Here's how the part is built. I have some questions about the finished solid (model axes, mm). A direction names the side the tool comes from. Coordinates: 2 decimals unless noted, no trailing zeros. Write each loop counter-clockwise with the first axis right and the second up, starting at its lowest first coordinate (ties: lowest second). Pieces come first, ordered by that corner, then holes. Notation, with made-up numbers: (30, -39) - (82, -39) arc R22 ccw to (82, -13) - close; hole circle Ø8 at (54, 37.5). An arc over 180 degrees is marked (long way). Answer in a Markdown table with one row per item. Add a question column.
Item 1: Which directions (+Z, -Z, +X, -X, +Y, -Y) give clear straight access to the entire face, cutting with the end or side of a thin tool? Please do faces 4 (the face through (-12, 2.28, -17.74)), 5 (the face through (-11, 0, 11)), 6 (the face through (-0.66, 11.409, 14.985)).
Item 2: We'd pull the mould along X, two halves only. Please class faces 1 (the face through (26.274, 2.465, -3.45)), 2 (the face through (23.636, 2.28, 0.215)), 3 (the face through (10, -13, 7)): +X half, -X half, draft (parallel to the pull), parting line (faces both ways), or undercut.
Item 3: Imagine slicing it at D-D (y = 1). Please give me the cut outline in (x, z), plus the area to 3 significant figures.
Item 4: Imagine slicing it at C-C (z = -6.5). Please give me the cut outline in (x, y).
Item 5: Imagine slicing it at A-A (x = 0). Please give me the cut outline in (y, z), plus the area to 3 significant figures.
Item 6: I'm going to push flat-ended pins straight in: pin 1 (12 mm diameter, centred on y = -9, z = 12.5, fed in from -X); pin 2 (2 mm diameter, centred on x = -11, z = -19.05, fed in from +Y); pin 3 (3 mm diameter, centred on x = 10.5, y = -6.5, fed in from +Z); pin 4 (5.5 mm diameter, centred on x = -11, z = 19.05, fed in from -Y). Where does each tip first touch, or does it pass through?
Item 7: Imagine slicing it at B-B (y = 11). Please give me the cut outline in (x, z), plus the area to 3 significant figures.
Item 8: If I drill on probe 1 along X at (y, z) = (2.55, 0); probe 2 along X at (y, z) = (0.5, -1.5); probe 3 along Y at (x, z) = (6.5, -17.5), over which ranges is the centre line in solid material (lowest first)? Write a range as from..to.
from build123d import *

# Parameters (mm, degrees)
SKETCH_1_R                   = 26.5
EXTRUDE_2_DEPTH              = 5
SKETCH_3_R                   = 15
EXTRUDE_3_DEPTH              = 13
EXTRUDE_START                = 13
SKETCH_4_R                   = 15
EXTRUDE_4_DEPTH              = 13
HOLE_WIZARD_M4_1_D           = 3.3
HOLE_WIZARD_M4_1_CSINK_D     = 4.05
HOLE_WIZARD_M4_1_CSINK_ANGLE = 90
PATTERN_CIRCULAR_1_COUNT     = 6
SKETCH_7_R                   = 11
CUT_EXTRUDE_1_DEPTH          = 31
SKETCH_8_R                   = 12
CUT_EXTRUDE_2_DEPTH          = 10


with BuildPart() as part:
    # 草图1 → 凸台-拉伸2 (new body)
    with BuildSketch(Plane(origin=(0, 0, 0), x_dir=(1, 0, 0), z_dir=(0, 1, 0))):
        with Locations(Location((0, 0, 0), (0, 0, 270))):
            Circle(SKETCH_1_R)
    extrude(amount=EXTRUDE_2_DEPTH)

    # 草图3 → 凸台-拉伸3 (add)
    with BuildSketch(Plane(origin=(0, 5, 0), x_dir=(1, 0, 0), z_dir=(0, 1, 0))):
        with Locations(Location((0, 0, 0), (0, 0, 90))):
            Circle(SKETCH_3_R)
    extrude(amount=EXTRUDE_3_DEPTH)

    # 草图4 → 凸台-拉伸4 (add)
    with BuildSketch(Plane.XZ.offset(EXTRUDE_START)):
        with Locations(Location((0, 0, 0), (0, 0, 270))):
            Circle(SKETCH_4_R)
    extrude(amount=-EXTRUDE_4_DEPTH)

    # M4 螺纹孔1 (through all)
    with Locations(Plane(origin=(22, 5, 0), x_dir=(0, 0, 1), z_dir=(0, 1, 0))):
        with Locations((0, 0)):
            hole_wizard_m4_1 = CounterSinkHole(HOLE_WIZARD_M4_1_D / 2, HOLE_WIZARD_M4_1_CSINK_D / 2, counter_sink_angle=HOLE_WIZARD_M4_1_CSINK_ANGLE)

    # 阵列(圆周)1: M4 螺纹孔1 ×6 about axis
    pattern_circular_1_axis = Axis((0, 0, 0), (0, 1, 0))
    for i in range(1, PATTERN_CIRCULAR_1_COUNT):
        add(hole_wizard_m4_1.rotate(pattern_circular_1_axis, i * 360 / PATTERN_CIRCULAR_1_COUNT), mode=Mode.SUBTRACT)

    # 草图7 → 切除-拉伸1 (cut)
    with BuildSketch(Plane(origin=(0, 18, 0), x_dir=(1, 0, 0), z_dir=(0, 1, 0))):
        with Locations(Location((0, 0, 0), (0, 0, 270))):
            Circle(SKETCH_7_R)
    extrude(amount=-CUT_EXTRUDE_1_DEPTH, mode=Mode.SUBTRACT)

    # 草图8 → 切除-拉伸2 (cut)
    with BuildSketch(Plane(origin=(0, 18, 0), x_dir=(1, 0, 0), z_dir=(0, 1, 0))):
        with Locations(Location((0, 0, 0), (0, 0, 270))):
            Circle(SKETCH_8_R)
    cut_extrude_2 = extrude(amount=-CUT_EXTRUDE_2_DEPTH, mode=Mode.SUBTRACT)

    # 镜向1: 切除-拉伸2 across plane
    add(cut_extrude_2.mirror(Plane.ZX.offset(2.5)), mode=Mode.SUBTRACT)


solid = part.part
Here are the results:
| question | item | result |
|---|---|---|
| 1 | face 4 | +Y, -Y |
| 1 | face 5 | -Y |
| 1 | face 6 | +Y |
| 2 | face 1 | parting line |
| 2 | face 2 | undercut |
| 2 | face 3 | draft |
| 3 | outline | circle Ø53 at (0, 0); hole circle Ø3.3 at (-22, 0); hole circle Ø3.3 at (-11, -19.05); hole circle Ø3.3 at (-11, 19.05); hole circle Ø22 at (0, 0); hole circle Ø3.3 at (11, -19.05); hole circle Ø3.3 at (11, 19.05); hole circle Ø3.3 at (22, 0) |
| 3 | area | 1,770 mm2 |
| 4 | outline | (-25.69, 0) - (-13.52, 0) - (-13.52, -13) - (-10.09, -13) - (-10.09, -3) - (-8.87, -3) - (-8.87, 8) - (-10.09, 8) - (-10.09, 18) - (-13.52, 18) - (-13.52, 5) - (-25.69, 5) - close; (8.87, -3) - (10.09, -3) - (10.09, -13) - (13.52, -13) - (13.52, 0) - (25.69, 0) - (25.69, 5) - (13.52, 5) - (13.52, 18) - (10.09, 18) - (10.09, 8) - (8.87, 8) - close |
| 5 | outline | (-13, -15) - (0, -15) - (0, -26.5) - (5, -26.5) - (5, -15) - (18, -15) - (18, -12) - (8, -12) - (8, -11) - (-3, -11) - (-3, -12) - (-13, -12) - close; (-13, 12) - (-3, 12) - (-3, 11) - (8, 11) - (8, 12) - (18, 12) - (18, 15) - (5, 15) - (5, 26.5) - (0, 26.5) - (0, 15) - (-13, 15) - close |
| 5 | area | 323 mm2 |
| 6 | pin 1 | stops at x = -13.52 |
| 6 | pin 2 | passes through |
| 6 | pin 3 | stops at z = 12 |
| 6 | pin 4 | stops at y = 0 |
| 7 | outline | circle Ø30 at (0, 0); hole circle Ø24 at (0, 0) |
| 7 | area | 254 mm2 |
| 8 | probe 1 | x = -26.5..-23.65, -20.35..-11, 11..20.35, 23.65..26.5 |
| 8 | probe 2 | x = -26.46..-22.69, -21.31..-10.9, 10.9..21.31, 22.69..26.46 |
| 8 | probe 3 | y = 0..5 |
